Geometry: final body of the model. Coordinates: model frame, mm. Face numbers are marked on the shaded views. A direction names the side the tool comes from. Coordinates: 2 decimals unless noted, no trailing zeros. Loops run counter-clockwise (first coordinate to the right, second up) from the corner with the lowest first, then second, coordinate; pieces in that order, holes last. Notation, with made-up numbers: (-34.5, 52) - (-24.5, 52) arc R12 cw to (-24.5, 68) - close; hole circle Ø10 at (-7, 88). An arc over 180 degrees is marked (long way). Answer in a Markdown table with one row per item.
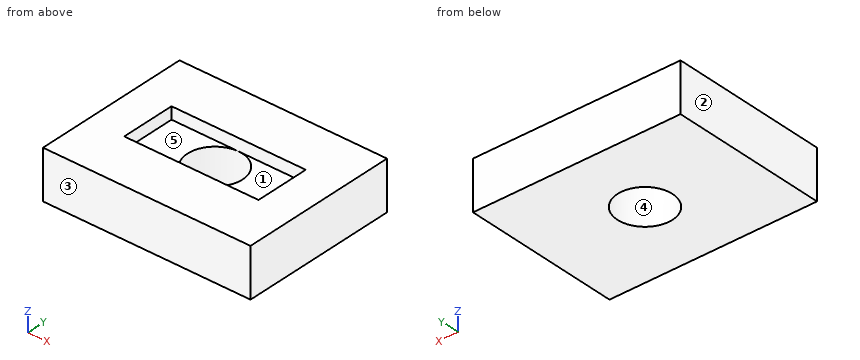
Autodesk Fusion 360 part; units mm, degrees
sketch "Sketch1" plane through (0, 0, 0) normal (0, 0, 1) x (1, 0, 0)
  circle A0 centre (0, 0) radius 4.5 construction
  line L0 (-11, 4.5) -> (11, 4.5) construction
  line L1 (11, 4.5) -> (11, -4.5) construction
  line L2 (11, -4.5) -> (-11, -4.5) construction
  line L3 (-11, -4.5) -> (-11, 4.5) construction
  line L4 (-17, 13) -> (17, 13)
  line L5 (17, 13) -> (17, -13)
  line L6 (17, -13) -> (-17, -13)
  line L7 (-17, -13) -> (-17, 13)
  dimension "d1" = 9
  dimension "d2" = 22
  dimension "d3" = 9
  dimension "d4" = 11
  dimension "d5" = 4.5
  dimension "d6" = 34
  dimension "d7" = 26
  dimension "d8" = 13
  dimension "d9" = 17
extrude "Extrude1" add sketch "Sketch1" along normal blind 10
sketch "Sketch2" plane through (0, 0, 10) normal (0, 0, 1) x (-1, 0, 0)
  line L0 (17, 13) -> (-17, 13)
  line L1 (-17, 13) -> (-17, -13)
  line L2 (-17, -13) -> (17, -13)
  line L3 (17, -13) -> (17, 13)
  line L4 (11, -4.5) -> (-11, -4.5)
  line L5 (-11, -4.5) -> (-11, 4.5)
  line L6 (-11, 4.5) -> (11, 4.5)
  line L7 (11, 4.5) -> (11, -4.5)
  dimension "d12" = 22
  dimension "d13" = 9
  dimension "d14" = 11
  dimension "d15" = 4.5
extrude "Extrude2" cut sketch "Sketch2" against normal blind 2 contours L4 L5 L6 L7
extrude "Extrude3" cut 1 faces at (-5.6667, 4.3333, 0) along direction (0, 0, 1) blind 2
sketch "Sketch3" plane through (0, 0, 8) normal (0, 0, 1) x (-1, 0, 0)
  line L0 (11, 4.5) -> (-11, 4.5)
  line L1 (-11, 4.5) -> (-11, -4.5)
  line L2 (-11, -4.5) -> (11, -4.5)
  line L3 (11, -4.5) -> (11, 4.5)
  circle A0 centre (0, 0) radius 4.5
  dimension "d20" = 9
extrude "Extrude4" cut sketch "Sketch3" against normal blind 26 contours A0
(1) First-contact query: pin 1 Ø2.5 at (x, y) = (-3, 0.5) entering from +Z. Flat tip, straight axial feed; report the tip coordinate or a pass-through.
Verdict:
| item | result |
|---|---|
| pin 1 | passes through |
(2) Cut plane A-A on y = -0.5. Output: boundary loops of the cut face in (x, z), then the cut area to 3 significant figures.
Verdict:
| item | result |
|---|---|
| outline | (-17, 2) - (-4.47, 2) - (-4.47, 8) - (-11, 8) - (-11, 10) - (-17, 10) - close; (4.47, 2) - (17, 2) - (17, 10) - (11, 10) - (11, 8) - (4.47, 8) - close |
| area | 174 mm² |
(3) Pull-direction query (Y, two-part tool) for the marked faces 1, 2 and 3; classes: pulls with the +Y half, pulls with the -Y half, needs draft (parallel to the pull), parting line crosses it, or undercut.
Verdict:
| item | result |
|---|---|
| face 1 | undercut |
| face 2 | needs draft |
| face 3 | pulls with the -Y half |
(4) Cut plane C-C on y = -4. Output: boundary loops of the cut face in (x, z).
Verdict:
| item | result |
|---|---|
| outline | (-17, 2) - (-2.06, 2) - (-2.06, 8) - (-11, 8) - (-11, 10) - (-17, 10) - close; (2.06, 2) - (17, 2) - (17, 10) - (11, 10) - (11, 8) - (2.06, 8) - close |
(5) Access query for the marked faces 4 and 5. Directions: +Z, -Z, +X, -X, +Y, -Y. A direction counts if a zero-diameter tool reaches every point of the face in a straight line with its end or side. Return the directions, or none.
Verdict:
| item | result |
|---|---|
| face 4 | +Z, -Z |
| face 5 | +Z |
(6) Ray query, probe 1 along X at (y, z) = (0, 3.3); probe 2 along Y at (x, z) = (0, 6.2); probe 3 along X at (y, z) = (-1, 5.5). Return the intervals inside material, ascending.
Verdict:
| item | result |
|---|---|
| probe 1 | x = -17 to -4.5, 4.5 to 17 |
| probe 2 | y = -13 to -4.5, 4.5 to 13 |
| probe 3 | x = -17 to -4.39, 4.39 to 17 |
(7) Cut plane B-B on z = 7. Output: boundary loops of the cut face in (x, y), then the cut area to 3 significant figures.
Verdict:
| item | result |
|---|---|
| outline | (-17, -13) - (17, -13) - (17, 13) - (-17, 13) - close; hole circle Ø9 at (0, 0) |
| area | 820 mm² |
